from build123d import *

# Parameters (mm, degrees)
F0_W     = 24.13
F0_H     = 24.13
F1_DEPTH = 24.13
F3_D     = 2.2606
F5_D     = 2.2606
F5_DEPTH = 12.066
F7_D     = 2.2606
F7_DEPTH = 12.066


with BuildPart() as f1:
    # F0 (on Top) → F1 (new body)
    with BuildSketch(Plane.XY):
        Rectangle(F0_W, F0_H)
    extrude(amount=F1_DEPTH)

    # F3 (through all)
    with Locations(Plane.XY.offset(24.13)):
        with Locations((0, 0)):
            Hole(F3_D / 2)

    # F5 (through all, one way)
    with BuildSketch(Plane.XZ):
        with Locations((0, 12.065)):
            Circle(F5_D / 2)
    extrude(amount=-F5_DEPTH, mode=Mode.SUBTRACT)

    # F7 (through all, one way)
    with BuildSketch(Plane.YZ):
        with Locations((0, 12.065)):
            Circle(F7_D / 2)
    extrude(amount=-F7_DEPTH, mode=Mode.SUBTRACT)


solid = f1.part
Here's how the part is built. I have some questions about the finished solid (model axes, mm). A direction names the side the tool comes from. Give positions to 0.01 mm unless a question says otherwise; leave off trailing zeros. Use one line per item in the form item = value. Start each with the question number.
1. If I drill on L1, parallel to Y at x = 0, z = 9.5 (3 decimals); L2, parallel to Z at x = -7.25, y = 0; L3, parallel to X at y = 0, z = 11.5 (3 decimals), over which ranges is the centre line in solid material (lowest first)?
2. On a 3-axis mill with a long thin cutter (end or side, diameter ignored), from which of +Z, -Z, +X, -X, +Y, -Y can I reach the whole of each face in a straight line? I mean faces 1 (the face through (-5.95, -1.13, 12.11)), 2 (the face through (0, 12.065, 9)), 3 (the face through (1.08, 5.95, 12.4)). Say none if no direction works.
3. Will this pin go through, and if not, where does the flat tip stop? pin 1 Ø2 at (x, y) = (9, 3) entering from -Z.
4. Thinking about a two-plate mould opening in Y: for faces 4 (the face through (0, -12.065, 12)), 5 (the face through (12.065, 0, 12)), 6 (the face through (0.897, -0.688, 11.896)), which applies, +Y half, -Y half, draft (parallel to the pull), parting line (faces both ways), or undercut?
Entries:
q1.L1 = -12.065 to -1.13, 1.13 to 12.065
q1.L2 = 0 to 10.93, 13.2 to 24.13
q1.L3 = 1.13 to 12.065
q2.face_1 = -X
q2.face_2 = +Z, -Z, +X, -X, +Y
q2.face_3 = +Y
q3.pin_1 = 0
q4.face_4 = -Y half
q4.face_5 = draft
q4.face_6 = undercut
